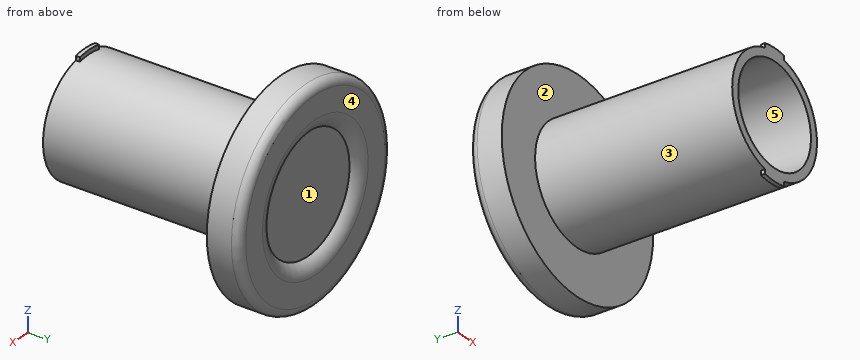
Autodesk Inventor part; units mm, degrees
ref_plane "YZ Plane" through (0, 0, 0) normal (1, 0, 0) x (0, 1, 0)
ref_plane "XZ Plane" through (0, 0, 0) normal (0, 1, 0) x (-1, 0, 0)
ref_plane "XY Plane" through (0, 0, 0) normal (0, 0, 1) x (1, 0, 0)
sketch "Sketch2" plane through (0, 0, 0) normal (1, 0, 0) x (0, 1, 0)
  line L0 (0, 0) -> (-4, 0)
  line L1 (-4, 0) -> (-4, -12.5)
  line L2 (-4, -12.5) -> (0, -12.5)
  line L3 (0, -12.5) -> (0, 0)
  line L4 (12.3022, 0) -> (-32.9738, 0) construction
  line L5 (-4, 0) -> (-28, 0)
  line L6 (-28, 0) -> (-28, -7)
  line L7 (-28, -7) -> (-4, -7)
  line L8 (-4, -7) -> (-4, 0)
  line L9 (-4, -6) -> (-28, -6)
  point P0 (-4, -7)
  dimension "d0" = 4
  dimension "d2" = 25
  dimension "d3" = 28
  dimension "d4" = 1
  dimension "d5" = 14
revolve "Revolution1" add sketch "Sketch2" angle 360 about axis through (0, 12.3022, 0) along (0, -1, 0) contours L3 L2 L1 L0 | L1 L7 L6 L9
sketch "Sketch3" plane through (0, 0, 0) normal (0, 1, 0) x (1, 0, 0)
  circle A0 centre (0, 0) radius 7
  dimension "d7" = 14
extrude "Extrusion1" cut sketch "Sketch3" against normal blind 1
fillet "Fillet1" radius 2 1 edges at (-7, 0, 0)
fillet "Fillet2" radius 1 1 edges at (0, 0, 12.5)
sketch "Sketch4" plane through (0, -28, 0) normal (0, -1, 0) x (1, 0, 0)
  circle A0 centre (0, 0) radius 7
  circle A1 centre (0, 0) radius 7
  line L0 (1.5845, 7.3307) -> (1.5845, 6.8183)
  line L1 (1.5845, -6.8183) -> (1.5845, -7.3307)
  line L2 (-1.5845, 7.3307) -> (-1.5845, 6.8183)
  line L3 (-1.5845, -6.8183) -> (-1.5845, -7.3307)
  circle A2 centre (0, 0) radius 11.5
  arc A3 (1.5845, 7.3307) -> (-1.5845, 7.3307) centre (0, 0) ccw
  arc A4 (-1.5845, -7.3307) -> (1.5845, -7.3307) centre (0, 0) ccw
  dimension "d13" = 1.5845
  dimension "d14" = 1.5845
  dimension "d15" = 1.5845
  dimension "d16" = 1.5845
extrude "Extrusion2" add sketch "Sketch4" against normal blind 0.5 contours A0 L2 A3 L0 | L1 A4 L3 A0
properties part number "BOTÃO"
CAD build for the part. Positions are in the model's coordinates, mm. Face numbers are marked on the shaded views. A direction names the side the tool comes from. Coordinates: 2 decimals unless noted, no trailing zeros. Order: outer loops, then holes, each group sorted by start corner. A loop starts at its lowest first (then second) coordinate and runs counter-clockwise, first axis right, second up. Notation, with made-up numbers: (11, 26.5) - (22, 26.5) arc R10 ccw to (22, 42.5) - close; hole circle Ø1 at (-7.75, 19). An arc over 180 degrees is marked (long way). Use a Markdown table: item, result. Add a question column.
(1) Saw through at B-B (x = 0). Give the cut face in (y, z).
(2) Saw through at A-A (z = 0). Give the cut face in (x, y), then the cut area to 3 significant figures.
(3) Saw through at C-C (y = -14.75). Give the cut face in (x, z).
(4) Pull direction X, two halves, no side cores. Call the marked faces 1, 2 and 3: +X half, -X half, draft (parallel to the pull), parting line (faces both ways), or undercut.
(5) Drill centre lines: line 1 along Z through (x, y) = (0.25, -21.5); line 2 along X through (y, z) = (-14.5, 0); line 3 along Y through (x, z) = (7, -8.5). Where is each one in solid material? Low to high. Write a range as [from, to].
(6) Which spindle directions (+Z, -Z, +X, -X, +Y, -Y) get a long thin tool onto all of the face, cutting with end or side? Do the marked faces 4 and 5. Say none if no direction does.
(7) Flat gauge pins, fed straight in: pin 1 (0.7 mm diameter, centred on x = 0.5, z = 7, fed in from +Y); pin 2 (3 mm diameter, centred on x = -5.5, y = -18.5, fed in from +Z); pin 3 (6 mm diameter, centred on x = 0, y = -24, fed in from -Z). Where does each tip first touch, or does it go through?
Solved:
| question | item | result |
|---|---|---|
| 1 | outline | (-28, -7.5) - (-27.5, -7.5) - (-27.5, -7) - (-4, -7) - (-4, -12.5) - (-1, -12.5) arc R1 ccw to (0, -11.5) - (0, -8.73) arc R2 ccw to (-1, -7) - (-1, 7) arc R2 ccw to (0, 8.73) - (0, 11.5) arc R1 ccw to (-1, 12.5) - (-4, 12.5) - (-4, 7) - (-27.5, 7) - (-27.5, 7.5) - (-28, 7.5) - (-28, 6) - (-4, 6) - (-4, -6) - (-28, -6) - close |
| 2 | outline | (-12.5, -4) - (-7, -4) - (-7, -28) - (-6, -28) - (-6, -4) - (6, -4) - (6, -28) - (7, -28) - (7, -4) - (12.5, -4) - (12.5, -1) arc R1 ccw to (11.5, 0) - (8.73, 0) arc R2 ccw to (7, -1) - (-7, -1) arc R2 ccw to (-8.73, 0) - (-11.5, 0) arc R1 ccw to (-12.5, -1) - close |
| 2 | area | 133 mm² |
| 3 | outline | circle Ø14 at (0, 0); hole circle Ø12 at (0, 0) |
| 4 | face 1 | undercut |
| 4 | face 2 | draft |
| 4 | face 3 | parting line |
| 5 | line 1 | z = [-7, -5.99], [5.99, 7] |
| 5 | line 2 | x = [-7, -6], [6, 7] |
| 5 | line 3 | y = [-4, 0] |
| 6 | face 4 | +Z, -Z, +X, -X, +Y |
| 6 | face 5 | -Y |
| 7 | pin 1 | stops at y = -0.54 |
| 7 | pin 2 | stops at z = 5.74 |
| 7 | pin 3 | stops at z = -7 |
